```python
from build123d import *

# Parameters (mm, degrees)
SKETCH_1_W               = 65
SKETCH_1_H               = 50
EXTRUDE_1_DEPTH          = 6
SKETCH_2_W               = 8
SKETCH_2_H               = 8
CUT_EXTRUDE_1_DEPTH      = 42.43971525
SKETCH_3_W               = 30
SKETCH_3_H               = 40
EXTRUDE_2_DEPTH          = 20
CUT_EXTRUDE_2_DEPTH      = 20
CUT_EXTRUDE_3_REACH      = 61.643
CUT_EXTRUDE_3_END_RADIUS = 6.5
SKETCH_5_R               = 3.5


with BuildPart() as part:
    # Эскиз1 → Бобышка-Вытянуть1 (new body)
    with BuildSketch(Plane.XY):
        Rectangle(SKETCH_1_W, SKETCH_1_H)
    extrude(amount=EXTRUDE_1_DEPTH)

    # Эскиз2 → Вырез-Вытянуть1 (cut, through all)
    with BuildSketch(Plane.XY.offset(6)):
        with Locations((-26.5, 19)):
            Rectangle(SKETCH_2_W, SKETCH_2_H)
        with Locations((26.5, -19)):
            Rectangle(SKETCH_2_W, SKETCH_2_H)
    extrude(amount=-CUT_EXTRUDE_1_DEPTH, mode=Mode.SUBTRACT)

    # Эскиз3 → Бобышка-Вытянуть2 (add)
    with BuildSketch(Plane.XY.offset(6)):
        with Locations((0, -5)):
            Rectangle(SKETCH_3_W, SKETCH_3_H)
    extrude(amount=EXTRUDE_2_DEPTH)

    # Эскиз4 → Вырез-Вытянуть2 (cut)
    with BuildSketch(Plane.XY.offset(26)):
        with BuildLine():
            Line((-5.5, 1.5), (5.5, 1.5))
            ThreePointArc((5.5, 1.5), (12, -5), (5.5, -11.5))
            Line((5.5, -11.5), (-5.5, -11.5))
            ThreePointArc((-5.5, -11.5), (-12, -5), (-5.5, 1.5))
        make_face()
    extrude(amount=-CUT_EXTRUDE_2_DEPTH, mode=Mode.SUBTRACT)

    # Вырез-Вытянуть3: up to this cylinder (the profile starts outside it)
    cut_extrude_3_end = Plane(origin=(-5.5, -5, 16), z_dir=(0, 0, 1)) * Cylinder(CUT_EXTRUDE_3_END_RADIUS, 137.286, mode=Mode.PRIVATE)
    # Эскиз5 → Вырез-Вытянуть3 (cut, up to the surface)
    with BuildSketch(Plane.ZY.offset(15), mode=Mode.PRIVATE) as cut_extrude_3_sk1:
        with Locations(Location((16, -5, 0), (0, 0, 270))):
            Circle(SKETCH_5_R)
    cut_extrude_3_tool1 = extrude(cut_extrude_3_sk1.sketch, amount=-CUT_EXTRUDE_3_REACH, mode=Mode.PRIVATE) - cut_extrude_3_end
    add(cut_extrude_3_tool1.solids().sort_by_distance((-15, -5, 16))[0], mode=Mode.SUBTRACT)


solid = part.part
```
Build history of the part. All positions in model axes, mm. A direction names the side the tool comes from. Coordinates: 2 decimals unless noted, no trailing zeros. Write each loop counter-clockwise with the first axis right and the second up, starting at its lowest first coordinate (ties: lowest second). Pieces come first, ordered by that corner, then holes.
1. Pull direction Y, two halves, no side cores. Call faces 1 (the flat face through (-27, 15, 3)), 2 (the flat face through (0, 17, 6)), 3 (the flat face through (0, -25, 10)): released by +Y, released by -Y, zero draft, split by the parting line, or undercut.
Answer block:
face 1: undercut
face 2: zero draft
face 3: released by -Y
2. Drop flat-ended pins along their axis: pin 1 (3 mm diameter, centred on x = -4, z = 23, fed in from +Y); pin 2 (3 mm diameter, centred on x = 6, y = 17, fed in from +Z); pin 3 (6 mm diameter, centred on y = -10, z = 12.5, fed in from +X). Give the stop position or say it passes through.
Answer block:
pin 1: stops at y = 15
pin 2: stops at z = 6
pin 3: stops at x = 15
3. Band-saw the part on B-B, the plane z = 24. Give the cut face in (x, y), and give its area (3 significant figures).
Answer block:
outline: (-15, -25) - (15, -25) - (15, 15) - (-15, 15) - close; hole (-5.5, -11.5) - (5.5, -11.5) arc R6.5 ccw to (5.5, 1.5) - (-5.5, 1.5) arc R6.5 ccw to start
area: 924 mm2
4. Band-saw the part on C-C, the plane x = 0.5. Give the cut face in (y, z).
Answer block:
outline: (-25, 0) - (25, 0) - (25, 6) - (15, 6) - (15, 26) - (1.5, 26) - (1.5, 6) - (-11.5, 6) - (-11.5, 26) - (-25, 26) - close
5. Drill centre lines: probe 1 along Z at (x, y) = (-13.3, -5); probe 2 along Y at (x, z) = (-12.2, 16); probe 3 along X at (y, z) = (9.5, 8). Where is each one in solid material? Low to high.
Answer block:
probe 1: z = 0 to 12.5, 19.5 to 26
probe 2: y = -25 to -8.5, -1.5 to 15
probe 3: x = -15 to 15
6. Band-saw the part on D-D, the plane z = 16. Give the cut face in (x, y).
Answer block:
outline: (-15, -25) - (15, -25) - (15, 15) - (-15, 15) - (-15, -1.5) - (-10.98, -1.5) arc R6.5 cw to (-5.5, 1.5) - (5.5, 1.5) arc R6.5 cw to (5.5, -11.5) - (-5.5, -11.5) arc R6.5 cw to (-10.98, -8.5) - (-15, -8.5) - close
7. 3-axis set-ups, long thin cutter, end or side, ignore diameter. For faces 4 (the flat face through (30.5, -19, 3)), 5 (the flat face through (0, -11.5, 16)), 6 (the cylindrical face through (-13.464, -8.233, 14.659)), 7 (the flat face through (0, 15, 16)): which of +Z, -Z, +X, -X, +Y, -Y reach the whole face in a straight line?
Answer block:
face 4: +Z, -Z
face 5: +Z
face 6: -X
face 7: +Z, +X, -X, +Y
8. Band-saw the part on A-A, the plane y = -5. Give the cut face in (x, z), and give its area (3 significant figures).
Answer block:
outline: (-32.5, 0) - (32.5, 0) - (32.5, 6) - (15, 6) - (15, 26) - (12, 26) - (12, 6) - (-12, 6) - (-12, 12.5) - (-15, 12.5) - (-15, 6) - (-32.5, 6) - close; (-15, 19.5) - (-12, 19.5) - (-12, 26) - (-15, 26) - close
area: 489 mm2
